```python
from build123d import *

# Parameters (mm, degrees)
SKETCH1_R           = 1
BOSS_EXTRUDE1_DEPTH = 8
BOSS_EXTRUDE2_DEPTH = 3


with BuildPart() as part:
    # Sketch1 → Boss-Extrude1 (new body)
    with BuildSketch(Plane.XY):
        with Locations((-63.49476159, 14.978708134)):
            Circle(SKETCH1_R)
    extrude(amount=BOSS_EXTRUDE1_DEPTH)

    # Sketch2 → Boss-Extrude2 (add)
    with BuildSketch(Plane(origin=(0, 0, 0), x_dir=(-1, 0, 0), z_dir=(0, 0, -1))):
        Polygon((63.49476159, 12.091956788), (65.99476159, 13.535332461), (65.99476159, 16.422083807), (63.49476159, 17.86545948), (60.99476159, 16.422083807), (60.99476159, 13.535332461), align=None)
    extrude(amount=BOSS_EXTRUDE2_DEPTH)


solid = part.part
```
Design review of the part built by this model. Coordinates are the model's own, in mm. A direction names the side the tool comes from. Coordinates: 2 decimals unless noted, no trailing zeros. Loops run counter-clockwise (first coordinate to the right, second up) from the corner with the lowest first, then second, coordinate; pieces in that order, holes last. Notation, with made-up numbers: (74, -2.5) - (126, -2.5) arc R25 cw to (126, 33.5) - close; hole circle Ø1 at (33, 41). An arc over 180 degrees is marked (long way). Use CSV: the item, a comma, the result in double quotes. Start each with the question number.
1) For pin 1 Ø2 at (x, z) = (-64.5, 2) entering from +Y; pin 2 Ø3 at (y, z) = (16.5, 3.5) entering from +X (3 decimals); pin 3 Ø3 at (y, z) = (16, 4) entering from -X, all flat-tipped, find the tip position at first contact; note any pin that passes through.
2) Wall thickness on L1, parallel to Z at x = -63.95, y = 12.6; L2, parallel to Y at x = -63.5, z = 3.75; L3, parallel to X at y = 15.05, z = 2.25: over which ranges is each line inside the solid? List them lowest first. Write a range as from..to.
3) Tool access review of faces 1 (the flat face through (-63.5, 13.7, 0)), 2 (the flat face through (-65.995, 15, -1)): name each direction out of +Z, -Z, +X, -X, +Y, -Y from which nothing blocks a thin tool from reaching the whole face with its end or side.
4) Consider section A-A on z = -0.25. Write out the cut boundary in (x, y), then the cut area to 3 significant figures.
5) Consider section C-C on x = -63.8. Write out the cut boundary in (y, z), then the cut area to 3 significant figures.
6) Consider section D-D on y = 13.75. Write out the cut boundary in (x, z), then the cut area to 3 significant figures.
7) Consider section B-B on y = 15.65. Write out the cut boundary in (x, z), then the cut area to 3 significant figures.
Geometry says:
1,pin 1,"y = 15.98"
1,pin 2,"x = -62.495"
1,pin 3,"x = -64.49"
2,L1,"-3..0"
2,L2,"13.98..15.98"
2,L3,"-64.49..-62.5"
3,face 1,"+Z"
3,face 2,"+Z, -Z, -X, +Y, -Y"
4,outline,"(-65.99, 13.54) - (-63.49, 12.09) - (-60.99, 13.54) - (-60.99, 16.42) - (-63.49, 17.87) - (-65.99, 16.42) - close"
4,area,"21.7 mm^2"
5,outline,"(12.27, -3) - (17.69, -3) - (17.69, 0) - (15.93, 0) - (15.93, 8) - (14.03, 8) - (14.03, 0) - (12.27, 0) - close"
5,area,"31.5 mm^2"
6,outline,"(-65.99, -3) - (-60.99, -3) - (-60.99, 0) - (-65.99, 0) - close"
6,area,"15.0 mm^2"
7,outline,"(-65.99, -3) - (-60.99, -3) - (-60.99, 0) - (-62.75, 0) - (-62.75, 8) - (-64.24, 8) - (-64.24, 0) - (-65.99, 0) - close"
7,area,"26.9 mm^2"
